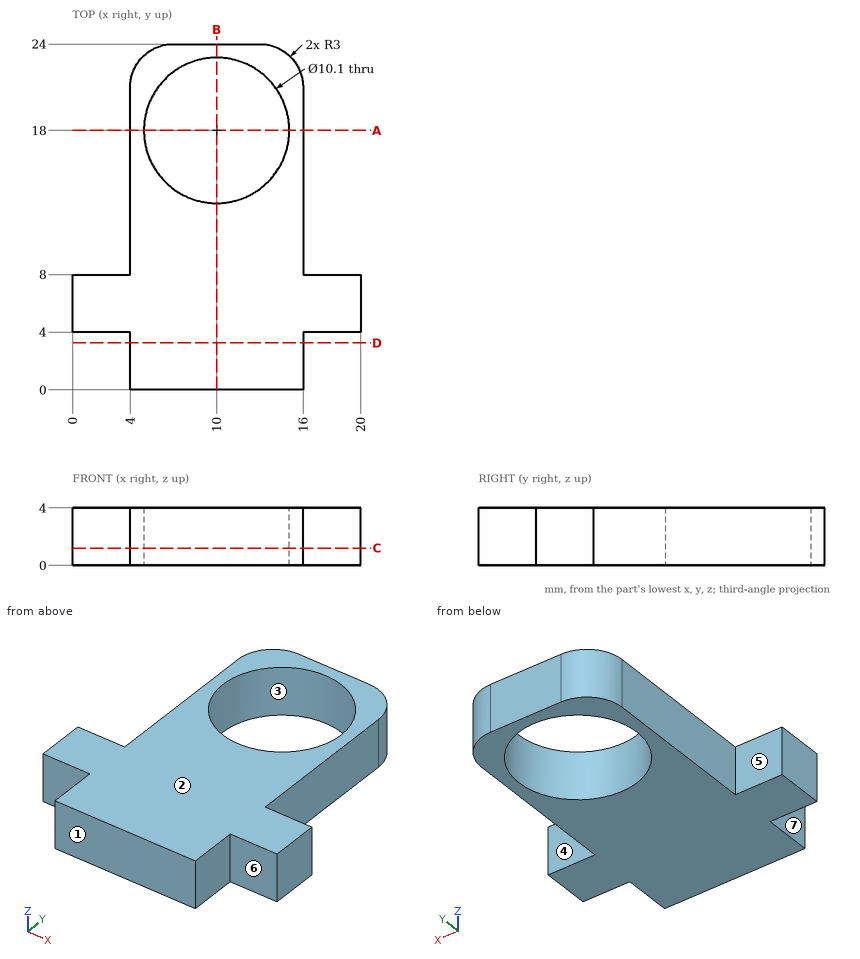
Drawing for the job (mm, zero at the part's lowest x, y, z). A direction names the side the tool comes from. Give positions to 0.01 mm unless a question says otherwise; leave off trailing zeros. Loops run counter-clockwise (first coordinate to the right, second up) from the corner with the lowest first, then second, coordinate; pieces in that order, holes last.
Item 1: Which spindle directions (+Z, -Z, +X, -X, +Y, -Y) get a long thin tool onto all of the face, cutting with end or side? Do the marked faces 5, 6 and 7. Say none if no direction does.
Check values:
face 5: +Z, -Z, -X, +Y
face 6: +Z, -Z, +X, -Y
face 7: +Z, -Z, -X, -Y
Item 2: Drop flat-ended pins along their axis: P1, Ø1.2, axis at y = 15, z = 3, coming from the +X side; P2, Ø1.2, axis at y = 2, z = 2.5, coming from the -X side; P3, Ø2, axis at x = 2, z = 1.5, coming from the +Y side. Give the stop position or say it passes through.
Check values:
P1: stops at x = 16
P2: stops at x = 4
P3: stops at y = 8
Item 3: Slice it at D-D (y = 3.25). Write the cut outline in (x, z), plus the area to 3 significant figures.
Check values:
outline: (4, 0) - (16, 0) - (16, 4) - (4, 4) - close
area: 48.0 mm2
Item 4: Slice it at C-C (z = 1.2). Write the cut outline in (x, y), plus the area to 3 significant figures.
Check values:
outline: (0, 4) - (4, 4) - (4, 0) - (16, 0) - (16, 4) - (20, 4) - (20, 8) - (16, 8) - (16, 21) arc R3 ccw to (13, 24) - (7, 24) arc R3 ccw to (4, 21) - (4, 8) - (0, 8) - close; hole circle Ø10.1 at (10, 18)
area: 236 mm2
Item 5: Mould opens along Y. For the marked faces 1, 2, 3 and 4 say: +Y half, -Y half, draft (parallel to the pull), parting line (faces both ways), or undercut.
Check values:
face 1: -Y half
face 2: draft
face 3: undercut
face 4: +Y half
Item 6: Drill centre lines: line 1 along Y through (x, z) = (10, 1.65); line 2 along Y through (x, z) = (19.25, 2.3); line 3 along X through (y, z) = (1.25, 0.35). Where is each one in solid material? Low to high.
Check values:
line 1: y = 0 to 12.95, 23.05 to 24
line 2: y = 4 to 8
line 3: x = 4 to 16
Item 7: Slice it at B-B (x = 10). Write the cut outline in (y, z).
Check values:
outline: (0, 0) - (12.95, 0) - (12.95, 4) - (0, 4) - close; (23.05, 0) - (24, 0) - (24, 4) - (23.05, 4) - close
Item 8: Slice it at A-A (y = 18). Write the cut outline in (x, z).
Check values:
outline: (4, 0) - (4.95, 0) - (4.95, 4) - (4, 4) - close; (15.05, 0) - (16, 0) - (16, 4) - (15.05, 4) - close
